Solid Edge part; units mm, degrees
sketch "Sketch1" plane through (0, 0, 0) normal (0, 0, 1) x (1, 0, 0)
  line L0 (0, 1.25) -> (10, 1.25)
  line L1 (10, 1.25) -> (10, 4.25)
  line L2 (10, 4.25) -> (0, 4.25)
  line L3 (0, 4.25) -> (0, 1.25)
  dimension "D1" = 10
  dimension "D2" = 10
extrude "Protrusion1" add sketch "Sketch1" along normal blind 10
mirror "Mirror1" about plane through (0, 0, 0) normal (0, -1, 0) of "Protrusion1"
sketch "Sketch2" plane through (3, -2.75, 0) normal (0, 0, -1) x (0, 1, 0)
  line L0 (-1.5, 7) -> (7, 7)
  line L1 (7, 7) -> (7, -3)
  line L2 (7, -3) -> (-1.5, -3)
  line L3 (-1.5, -3) -> (-1.5, 7)
extrude "Extrusionsausprägung_2" add sketch "Sketch2" along normal blind 15
hole "Bohrung_1" at (3.5, 4.25, 6) direction (0, -1, 0) diameter 2.459 end through all
fillet "Verrundung_1" radius 2.5 2 edges at (0, -2.75, 10) (0, 2.75, 10)
sketch "Sketch3" plane through (5, 4.25, 0) normal (0, 1, 0) x (-1, 0, 0)
  line L0 (-2.04, -8.976) -> (-2.04, 16.024)
  line L1 (-2.04, -8.976) -> (-2.04, -11.4934)
  dimension "D1" = 2.04
extrude "Extrusionsausschnitt_1" cut sketch "Sketch3" against normal blind 92.5 material side at (7.09, 4.25, 3.524)
hole "Bohrung_2" at (7.04, 0, -10.55) direction (-1, 0, 0) diameter 2.459 end up to next
fillet "Verrundung_2" radius 1.5 2 edges at (7.04, -2.75, 10) (7.04, 2.75, 10)
Geometry: final body of the model. Coordinates: model frame, mm. A direction names the side the tool comes from. Give positions to 0.01 mm unless a question says otherwise; leave off trailing zeros. Loops run counter-clockwise (first coordinate to the right, second up) from the corner with the lowest first, then second, coordinate; pieces in that order, holes last. Notation, with made-up numbers: (57, 89.25) - (110, 89.25) arc R15 ccw to (110, 117.25) - close; hole circle Ø5 at (74.25, 68). An arc over 180 degrees is marked (long way). Answer as CSV lines item,"result". Start each with the question number.
1. Ray query, L1, parallel to Y at x = 1.5, z = -10.55; L2, parallel to Z at x = 5.5, y = 0; L3, parallel to X at y = -2.95, z = 6. Return the intervals inside material, ascending.
2. Draft query along Y for faces 3 (the face through (0, 0, -4)), 4 (the face through (3, 0, 0)), 5 (the face through (3, -4.25, -2)), 6 (the face through (3, 1.25, 4)). Return one class per face: released by +Y, released by -Y, zero draft, split by the parting line, or undercut.
3. Section A-A, the plane z = 2.5. Return loops of the section in (x, y).
4. Section C-C, the plane y = 0. Return loops of the section in (x, z), plus the area to 3 significant figures.
5. Section B-B, the plane x = 3.5. Return loops of the section in (y, z).
6. Section D-D, the plane z = 6. Return loops of the section in (x, y), plus the area to 3 significant figures.
7. Reachability of faces 1 (the face through (4.4, -1.25, 4.9)), 2 (the face through (4, -3, 10)) from +Z, -Z, +X, -X, +Y, -Y: full face, straight path, thin tool, end or side. Return the list, or none.
8. Pin query (flat end, axial travel): P1, Ø2, axis at x = 1, y = 1.5, coming from the +Z side; P2, Ø1.2, axis at x = 5, y = 0.5, coming from the +Z side. Return the tip coordinate at first contact, or that it passes through.
Answers:
1,L1,"y = -4.25 to -1.23, 1.23 to 4.25"
1,L2,"z = -15 to -11.78, -9.32 to 0"
1,L3,"x = 0 to 2.27, 4.73 to 7.04"
2,face 3,"zero draft"
2,face 4,"undercut"
2,face 5,"released by -Y"
2,face 6,"undercut"
3,outline,"(0, -4.25) - (7.04, -4.25) - (7.04, -1.25) - (0, -1.25) - close; (0, 1.25) - (7.04, 1.25) - (7.04, 4.25) - (0, 4.25) - close"
4,outline,"(0, -15) - (7.04, -15) - (7.04, -11.78) - (0, -11.78) - close; (0, -9.32) - (7.04, -9.32) - (7.04, 0) - (0, 0) - close"
4,area,"88.3 mm2"
5,outline,"(-4.25, -15) - (4.25, -15) - (4.25, 4.77) - (1.25, 4.77) - (1.25, 0) - (-1.25, 0) - (-1.25, 4.77) - (-4.25, 4.77) - close; (-4.25, 7.23) - (-1.25, 7.23) - (-1.25, 10) - (-4.25, 10) - close; (1.25, 7.23) - (4.25, 7.23) - (4.25, 10) - (1.25, 10) - close; hole circle Ø2.46 at (0, -10.55)"
6,outline,"(0, -4.25) - (2.27, -4.25) - (2.27, -1.25) - (0, -1.25) - close; (0, 1.25) - (2.27, 1.25) - (2.27, 4.25) - (0, 4.25) - close; (4.73, -4.25) - (7.04, -4.25) - (7.04, -1.25) - (4.73, -1.25) - close; (4.73, 1.25) - (7.04, 1.25) - (7.04, 4.25) - (4.73, 4.25) - close"
6,area,"27.5 mm2"
7,face 1,"+Z, +X, -X"
7,face 2,"+Z, +X, -X, +Y, -Y"
8,P1,"stops at z = 9.95"
8,P2,"stops at z = 0"
